Autodesk Inventor part; units mm, degrees
ref_plane "YZ Plane" through (0, 0, 0) normal (1, 0, 0) x (0, 1, 0)
ref_plane "XZ Plane" through (0, 0, 0) normal (0, 1, 0) x (-1, 0, 0)
ref_plane "XY Plane" through (0, 0, 0) normal (0, 0, 1) x (1, 0, 0)
sketch "Эскиз1" plane through (0, 0, 0) normal (0, 0, 1) x (1, 0, 0)
  circle A0 centre (0, 0) radius 3.25
  circle A1 centre (0, 0) radius 4.5
  dimension "d0" = 6.5
  dimension "d1" = 9
extrude "Выдавливание1" add sketch "Эскиз1" along normal blind 5.25
sketch "Эскиз2" plane through (0, 0, 0) normal (0, 0, -1) x (-1, 0, 0)
  circle A0 centre (0, 0) radius 5.5
  dimension "d4" = 11
loft "Лофт1" add profiles "Эскиз2" section 2 edges at (-4.5, 0, 5.25)
sketch "Эскиз4" plane through (0, 0, 0) normal (0, 0, -1) x (-1, 0, 0)
  circle A0 centre (0, 0) radius 3.25
  dimension "d10" = 6.5
extrude "Выдавливание2" cut sketch "Эскиз4" against normal through all
sketch "Эскиз5" plane through (0, 0, 0) normal (0, 0, -1) x (-1, 0, 0)
  circle A0 centre (-8.8669, 1.5421) radius 2.1
  circle A1 centre (-1.5421, -8.8669) radius 2.1
  circle A2 centre (1.5421, 8.8669) radius 2.1
  circle A3 centre (8.8669, -1.5421) radius 2.1
  circle A4 centre (0, 0) radius 13.5
  circle A5 centre (0, 0) radius 3.25
  dimension "d13" = 27
extrude "Выдавливание3" add sketch "Эскиз5" against normal blind 4
fillet "Сопряжение1" radius 2 1 edges at (4.7381, 0, 4)
chamfer "Фаска1" distance 2 angle 45 4 edges at (0.5579, 8.8669, 4) (10.9669, 1.5421, 4) (-6.7669, -1.5421, 4) (3.6421, -8.8669, 4)
sketch "Эскиз6" plane through (0, 0, 0) normal (0, 0, -1) x (-1, 0, 0)
  circle A0 centre (0, 0) radius 13.5
  circle A1 centre (8.8669, -1.5421) radius 2.1
  circle A2 centre (1.5421, 8.8669) radius 2.1
  circle A3 centre (-1.5421, -8.8669) radius 2.1
  circle A4 centre (-8.8669, 1.5421) radius 2.1
  circle A5 centre (0, 0) radius 3.25
extrude "Выдавливание4" cut sketch "Эскиз6" against normal blind 2
sketch "Эскиз7" plane through (0, 0, 2) normal (0, 0, -1) x (-1, 0, 0)
  circle A0 centre (0, 0) radius 13.5
  circle A1 centre (0, 0) radius 3.25
  arc A2 (-7.0308, 2.5612) -> (-7.4827, -0.0371) centre (-8.8669, 1.5421) ccw
  arc A3 (-2.5612, -7.0308) -> (0.0371, -7.4827) centre (-1.5421, -8.8669) ccw
  arc A4 (2.5612, 7.0308) -> (-0.0371, 7.4827) centre (1.5421, 8.8669) ccw
  arc A5 (7.0308, -2.5612) -> (7.4827, 0.0371) centre (8.8669, -1.5421) ccw
extrude "Выдавливание5" add sketch "Эскиз7" against normal blind 2 contours A1
properties part number "втулка для крепл" material "Пластик ПЭТ"
For this review, take the finished solid that the model builds, in its own axes (mm). A direction names the side the tool comes from. Coordinates: 2 decimals unless noted, no trailing zeros. Return JSON: item names as keys, results as strings.
1. For pin 1 Ø1.5 at (x, z) = (1.5, 2.5) entering from -Y; pin 2 Ø1.5 at (x, z) = (-6, 3) entering from -Y; pin 3 Ø8 at (x, y) = (7.5, -7.5) entering from +Z, all flat-tipped, find the tip position at first contact; note any pin that passes through.
Answer block:
{"pin 1": "y = -13.48", "pin 2": "y = -12.44", "pin 3": "z = 4"}
2. The part is to be moulded in two halves that separate along Y. For faces 3 (the cylindrical face through (2.93, -13.18, 2.99)), 4 (the flat face through (3, -2, 5.25)), 5 (the flat face through (0, 0, 4)), say which applies: +Y half, -Y half, draft (parallel to the pull), parting line (faces both ways), or undercut.
Answer block:
{"face 3": "parting line", "face 4": "draft", "face 5": "undercut"}
3. We need section A-A on z = 2.55. State how many separate pieces and enclosed holes the cut face has, and give its area (3 significant figures).
Answer block:
{"separate pieces": "1", "enclosed holes": "4", "area": "485 mm²"}
4. For line 1 (X direction, y = -0.5, z = 2.4); line 2 (X direction, y = -2.75, z = 3.2); line 3 (Y direction, x = 8.25, z = 3.75), list the stretches that pass through material, from the lowest coordinate up. Write a range as from..to.
Answer block:
{"line 1": "-13.49..-11.14, -6.67..7.42, 10.31..13.49", "line 2": "-13.22..-11.94, -5.83..13.22", "line 3": "-10.69..-2.26, 5.34..10.69"}
5. Machinability: for faces 1 (the flat face through (0, 0, 2)), 2 (the cylindrical face through (2.579, -1.978, 4.616)), which of the approach directions +Z, -Z, +X, -X, +Y, -Y give a long, thin tool a straight path to every point of the face, cutting with its end or side? Answer none if there is none.
Answer block:
{"face 1": "-Z, +X, -X, +Y, -Y", "face 2": "+Z"}
